For this review, take the finished solid that the model builds, in its own axes (mm). A direction names the side the tool comes from. Round coordinates to 2 decimals unless told otherwise and drop trailing zeros. Loops run counter-clockwise (first coordinate to the right, second up) from the corner with the lowest first, then second, coordinate; pieces in that order, holes last.
```python
from build123d import *

# Parameters (mm, degrees)
F0_R            = 13.5
F1_DEPTH        = 15
F2_R            = 10
F3_DEPTH        = 10
F4_R            = 5
F5_DEPTH        = 25.001
F7_DEPTH        = 25.001
F7_COPIES_COUNT = 25


# Not quite as in the source:
# - a pattern or mirror of a feature is missing from the dataset's text; its kind, count and spacing are read off the source's solid


with BuildPart() as f1:
    # F0 (on Top) → F1 (new body)
    with BuildSketch(Plane.XY):
        Circle(F0_R)
    extrude(amount=F1_DEPTH)

    # F2 (on face) → F3 (join)
    with BuildSketch(Plane.XY.offset(15)):
        Circle(F2_R)
    extrude(amount=F3_DEPTH)

    # F4 (on face) → F5 (cut, through all)
    with BuildSketch(Plane.XY.offset(25)):
        Circle(F4_R)
    extrude(amount=-F5_DEPTH, mode=Mode.SUBTRACT)

    # F6 (on face) → F7 (cut, through all)
    with BuildSketch(Plane(origin=(0, 0, 0), x_dir=(1, 0, 0), z_dir=(0, 0, -1))):
        with BuildLine():
            Line((-13.3188989942, -2.2038442736), (-11.1612903898, -1.4099988776))
            Line((-11.1612903898, -1.4099988776), (-11.2378712938, -0.5222535625))
            Line((-11.2378712938, -0.5222535625), (-13.5, 0))
            ThreePointArc((-13.5, 0), (-13.4546485726, -1.1056363729), (-13.3188989942, -2.2038442736))
        make_face()
    f7 = extrude(amount=-F7_DEPTH, mode=Mode.SUBTRACT)

    # F7_copies: F7 ×25 about axis
    f7_copies_axis = Axis((0, 0, 0), (0, 0, 1))
    for i in range(1, F7_COPIES_COUNT):
        add(f7.rotate(f7_copies_axis, i * 360 / F7_COPIES_COUNT), mode=Mode.SUBTRACT)


solid = f1.part
```
(1) Insertion check: pin 1 Ø4 at (x, z) = (2.5, 9) entering from -Y; pin 2 Ø5 at (x, z) = (-4, 7.5) entering from -Y. Each pin has a flat end and moves straight along its axis. Give the tip position at first contact, or say it passes through.
(2) For L1, parallel to Y at x = 0, z = 13; L2, parallel to Z at x = -7, y = 9.25; L3, parallel to X at y = 8.25, z = 1.5, list the stretches that pass through material, from the lowest coordinate up.
(3) Add section A-A (z = 22). Give the boundary of the cut face in (x, y).
(4) For faces 4 (the flat face through (0.516, -12.378, 7.395)), 5 (the flat face through (11.931, -3.334, 7.395)), 6 (the flat face through (-2.54, 10.95, 7.4)), 7 (the flat face through (9.838, -7.475, 7.395)), list the 3-axis set-ups (+Z, -Z, +X, -X, +Y, -Y) from which the entire face can be reached by the end or side of a thin tool; tool diameter is ignored.
(5) The part is to be moulded in two halves that separate along Y. For faces 1 (the cylindrical face through (-13.21, 2.79, 7.4)), 2 (the flat face through (-11.419, 4.803, 7.395)), 3 (the flat face through (-5.511, -11.095, 7.395)), say which applies: pulls with the +Y half, pulls with the -Y half, needs draft (parallel to the pull), parting line crosses it, or undercut.
Outcome:
1. pin 1: stops at y = -13.26
1. pin 2: stops at y = -13.15
2. L1: y = -13.5 to -5, 5 to 11.24
2. L2: z = 0 to 15
2. L3: x = -10.52 to -8.14, -7.64 to 7.64, 9.14 to 10.69
3. outline: circle Ø20 at (0, 0); hole circle Ø10 at (0, 0)
4. face 4: +Z, -Z, -Y
4. face 5: +Z, -Z, +X
4. face 6: +Z, -Z, +Y
4. face 7: +Z, -Z
5. face 1: pulls with the +Y half
5. face 2: undercut
5. face 3: pulls with the -Y half
